Model file for the job. Use its own axes, mm. A direction names the side the tool comes from. Give positions to 0.01 mm unless a question says otherwise; leave off trailing zeros. Order: outer loops, then holes, each group sorted by start corner. A loop starts at its lowest first (then second) coordinate and runs counter-clockwise, first axis right, second up. Notation, with made-up numbers: M 23,72.5 L 73,72.5 A23 cw 73,111.5 Z; hole C 38,59.5 d3. An arc over 180 degrees is marked long. Return JSON: item names as keys, results as strings. Group by question number.
1. 3-axis set-ups, long thin cutter, end or side, ignore diameter. For faces 1 (the face through (-1, 38, 0)), 2 (the face through (0, 11, 3)): which of +Z, -Z, +X, -X, +Y, -Y reach the whole face in a straight line?
2. Slice it at A-A on y = 75. List the corners of the cut face in (x, z).
3. Slice it at B-B on x = 0. List the corners of the cut face in (y, z), then the cut area to 3 significant figures.
4. Slice it at C-C on z = 3.8. List the corners of the cut face in (x, y), then the cut area to 3 significant figures.
5. Slice it at D-D on x = -28.5. List the corners of the cut face in (y, z).
6. Two-plate mould, pull along Y, no slides. Class faces 3 (the face through (-1, 0, 3)), 4 (the face through (-50, 29, 3)), 5 (the face through (-22.5, 9, 3)): released by +Y, released by -Y, zero draft, split by the parting line, or undercut.
7. Wall check: probe 1 along Y at (x, z) = (0, 4.3); probe 2 along X at (y, z) = (75, 3.15); probe 3 along X at (y, z) = (72.5, 1.1). Give the ranges that are in metal, low to high. Write a range as [from, to].
8. Pin check, flat tip, straight feed: pin 1 (2 mm diameter, centred on x = -11.5, z = 4.5, fed in from +Y). Stop position of the tip, or through.
Autodesk Inventor part; units mm, degrees
ref_plane "Work Plane1" through (0, 0, 6) normal (1, 0, 0) x (0, 0, -1)
ref_plane "YZ Plane" through (0, 0, 0) normal (1, 0, 0) x (0, 1, 0)
ref_plane "XZ Plane" through (0, 0, 0) normal (0, 1, 0) x (-1, 0, 0)
sketch "Sketch1" plane through (0, 0, 0) normal (0, 0, 1) x (1, 0, 0)
  line L0 (-50, 0) -> (50, 0)
  line L1 (50, 0) -> (50, 55)
  line L2 (10, 95) -> (-10, 95)
  line L3 (-50, 55) -> (-50, 0)
  line L4 (-50, 55) -> (-10, 95)
  line L5 (50, 55) -> (10, 95)
  point P0 (0, 0)
  point P1 (50, 95)
  point P2 (-50, 95)
  point P3 (0, 0)
  dimension "d2" = 95
  dimension "d3" = 100
  dimension "d4" = 40
  dimension "d5" = 40
  dimension "d6" = 40
  dimension "d7" = 40
extrude "Plate1" add sketch "Sketch1" along normal blind 6
hole "Hole1" at (0, 75, 6) direction (0, 0, -1) diameter 15 depth 6 tip angle 118
fillet "Corner Round1" radius 5 6 edges at (-50, 0, 3) (50, 0, 3) (50, 55, 3) (10, 95, 3) (-10, 95, 3) (-50, 55, 3)
ref_plane "Work Plane1" through (0, 0, 6) normal (1, 0, 0) x (0, 0, -1)
sketch "Sketch2" plane through (-45, 0, 6) normal (0, 0, 1) x (1, 0, 0)
  circle A0 centre (45, 75) radius 7.5
  line L0 (22.5, 11) -> (67.5, 11)
  line L1 (67.5, 11) -> (67.5, 7)
  line L2 (67.5, 7) -> (22.5, 7)
  line L3 (22.5, 7) -> (22.5, 11)
  point P0 (0, 0)
  dimension "d19" = 4
  dimension "d20" = 45
  dimension "d21" = 7
  dimension "d22" = 22.5
extrude "Cut1" cut sketch "Sketch2" against normal blind 6 contours L0 L1 L2 L3
equation "\"d16\" = Thickness"
equation "\"d23\" = Thickness"
equation "\"BendReliefWidth\" = Thickness"
equation "\"CornerReliefSize\" = 4 * Thickness"
equation "\"MinimumRemnant\" = 2 * Thickness"
equation "\"TransitionRadius\" = BendRadius"
equation "\"d8\" = BendRadius"
equation "\"JacobiRadiusSize\" = Thickness"
equation "\"GapSize\" = Thickness"
properties part number "voetplaat poot" material "Steel, Mild"
Result:
{
 "1": {"face 1": "-Z, +X, -X, +Y, -Y", "face 2": "+Z, -Z"},
 "2": {"outline": "M -30,0 L -7.5,0 L -7.5,6 L -30,6 Z; M 7.5,0 L 30,0 L 30,6 L 7.5,6 Z"},
 "3": {"outline": "M 0,0 L 7,0 L 7,6 L 0,6 Z; M 11,0 L 67.5,0 L 67.5,6 L 11,6 Z; M 82.5,0 L 95,0 L 95,6 L 82.5,6 Z", "area": "456 mm2"},
 "4": {"outline": "M -50,5 A5 ccw -45,0 L 45,0 A5 ccw 50,5 L 50,52.93 A5 ccw 48.54,56.46 L 11.46,93.54 A5 ccw 7.93,95 L -7.93,95 A5 ccw -11.46,93.54 L -48.54,56.46 A5 ccw -50,52.93 Z; hole M -22.5,7 L 22.5,7 L 22.5,11 L -22.5,11 Z; hole C 0,75 d15", "area": "7,530 mm2"},
 "5": {"outline": "M 0,0 L 76.5,0 L 76.5,6 L 0,6 Z"},
 "6": {"face 3": "released by -Y", "face 4": "zero draft", "face 5": "undercut"},
 "7": {"probe 1": "y = [0, 7], [11, 67.5], [82.5, 95]", "probe 2": "x = [-30, -7.5], [7.5, 30]", "probe 3": "x = [-32.5, -7.07], [7.07, 32.5]"},
 "8": {"pin 1": "stops at y = 94.29"}
}
